Input: part model. Units: mm. Frame: model coordinates. Coordinates: 2 decimals unless noted, no trailing zeros. Order: outer loops, then holes, each group sorted by start corner. A loop starts at its lowest first (then second) coordinate and runs counter-clockwise, first axis right, second up.
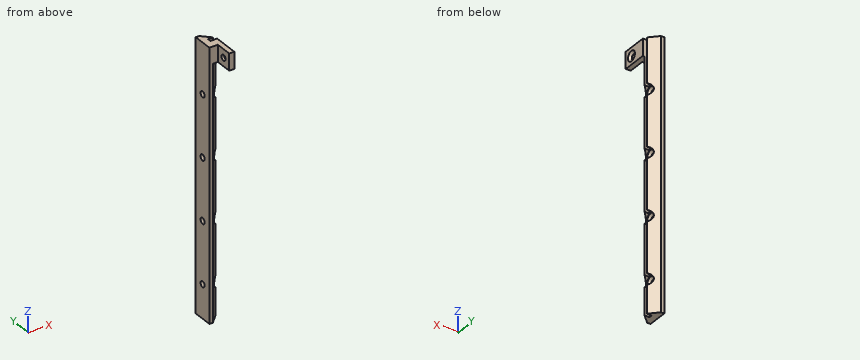
from build123d import *

# Parameters (mm, degrees)
BOSS_EXTRUDE1_DEPTH                            = 75
SKETCH5_R                                      = 1.75
CUT_EXTRUDE1_DEPTH                             = 2
CSK_FOR_0_FLAT_HEAD_MACHINE_SCREW2_D           = 1.778
CSK_FOR_0_FLAT_HEAD_MACHINE_SCREW2_DEPTH       = 3.302
CSK_FOR_0_FLAT_HEAD_MACHINE_SCREW2_CSINK_D     = 3.0226
CSK_FOR_0_FLAT_HEAD_MACHINE_SCREW2_CSINK_ANGLE = 82
CSK_FOR_0_FLAT_HEAD_MACHINE_SCREW2_TIP         = 0.53416509
CHAMFER1_SIZE                                  = 3
SKETCH6_W                                      = 1.5
SKETCH6_H                                      = 5
BOSS_EXTRUDE2_DEPTH                            = 5
CSK_FOR_0_FLAT_HEAD_MACHINE_SCREW1_D           = 1.778
CSK_FOR_0_FLAT_HEAD_MACHINE_SCREW1_DEPTH       = 3.302
CSK_FOR_0_FLAT_HEAD_MACHINE_SCREW1_CSINK_D     = 3.0226
CSK_FOR_0_FLAT_HEAD_MACHINE_SCREW1_CSINK_ANGLE = 82
CSK_FOR_0_FLAT_HEAD_MACHINE_SCREW1_TIP         = 0.53416509


with BuildPart() as part:
    # Sketch1 → Boss-Extrude1 (new body)
    with BuildSketch(Plane.XY):
        Polygon((-2, -3), (2, -3), (2, -0.5), (0, -0.5), (0, 0.5), (2, 0.5), (2, 3), (-2, 3), align=None)
    extrude(amount=BOSS_EXTRUDE1_DEPTH)

    # Sketch5 → Cut-Extrude1 (cut)
    with BuildSketch(Plane(origin=(2, 0, 0), x_dir=(0, 0, -1), z_dir=(1, 0, 0))):
        with Locations((-65, 0)):
            Circle(SKETCH5_R)
        with Locations((-46.66667, 0)):
            Circle(SKETCH5_R)
        with Locations((-28.33334, 0)):
            Circle(SKETCH5_R)
        with Locations((-10.00001, 0)):
            Circle(SKETCH5_R)
    extrude(amount=-CUT_EXTRUDE1_DEPTH, mode=Mode.SUBTRACT)

    # CSK for #0 Flat Head Machine Screw2
    with Locations(Plane(origin=(0, 0, 0), x_dir=(0, 0, -1), z_dir=(1, 0, 0))):
        with Locations((-65, 0), (-10.00001, 0), (-46.66667, 0), (-28.33334, 0)):
            CounterSinkHole(CSK_FOR_0_FLAT_HEAD_MACHINE_SCREW2_D / 2, CSK_FOR_0_FLAT_HEAD_MACHINE_SCREW2_CSINK_D / 2, depth=CSK_FOR_0_FLAT_HEAD_MACHINE_SCREW2_DEPTH, counter_sink_angle=CSK_FOR_0_FLAT_HEAD_MACHINE_SCREW2_CSINK_ANGLE)
            with Locations((0, 0, -(CSK_FOR_0_FLAT_HEAD_MACHINE_SCREW2_DEPTH + CSK_FOR_0_FLAT_HEAD_MACHINE_SCREW2_TIP / 2))):  # 118° drill point
                Cone(0, CSK_FOR_0_FLAT_HEAD_MACHINE_SCREW2_D / 2, CSK_FOR_0_FLAT_HEAD_MACHINE_SCREW2_TIP, mode=Mode.SUBTRACT)

    # Chamfer1
    # the kernel refuses this chamfer: 3 mm, written as the material it takes off along each edge
    with BuildSketch(Plane(origin=(2, -3, -7.715048964), x_dir=(-0.9996219169112968, -0.027495876610586348, 0), z_dir=(0, 0, 1))) as chamfer1_piece_1:
        Polygon((CHAMFER1_SIZE * 0.999621916911, -CHAMFER1_SIZE * 0.0274958766106), (-CHAMFER1_SIZE * 0.0274958766106, -CHAMFER1_SIZE * 0.999621916911), (0, 0), align=None)
    extrude(amount=90.430097928, mode=Mode.SUBTRACT)
    with BuildSketch(Plane(origin=(2, 3, -7.715048964), x_dir=(-0.9996219169112968, 0.027495876610586348, 0), z_dir=(0, 0, 1))) as chamfer1_piece_2:
        Polygon((CHAMFER1_SIZE * 0.999621916911, CHAMFER1_SIZE * 0.0274958766106), (-CHAMFER1_SIZE * 0.0274958766106, CHAMFER1_SIZE * 0.999621916911), (0, 0), align=None)
    extrude(amount=90.430097928, mode=Mode.SUBTRACT)

    # Sketch6 → Boss-Extrude2 (add)
    with BuildSketch(Plane.XY.offset(75)):
        Polygon((-2, 3), (-2, -3), (-1, -3), (1.5, -0.5), (0, -0.5), (0, 0.5), (1.5, 0.5), (-1, 3), align=None)
        Polygon((1.5, -0.5), (-1, -3), (0.5, -3), (2, -3), (2, -0.5), align=None)
        with Locations((1.25, -5.5)):
            Rectangle(SKETCH6_W, SKETCH6_H)
    extrude(amount=BOSS_EXTRUDE2_DEPTH)

    # CSK for #0 Flat Head Machine Screw1
    with Locations(Plane(origin=(2, 0, 0), x_dir=(0, 0, -1), z_dir=(1, 0, 0))):
        with Locations((-77.5, -5.5)):
            CounterSinkHole(CSK_FOR_0_FLAT_HEAD_MACHINE_SCREW1_D / 2, CSK_FOR_0_FLAT_HEAD_MACHINE_SCREW1_CSINK_D / 2, depth=CSK_FOR_0_FLAT_HEAD_MACHINE_SCREW1_DEPTH, counter_sink_angle=CSK_FOR_0_FLAT_HEAD_MACHINE_SCREW1_CSINK_ANGLE)
            with Locations((0, 0, -(CSK_FOR_0_FLAT_HEAD_MACHINE_SCREW1_DEPTH + CSK_FOR_0_FLAT_HEAD_MACHINE_SCREW1_TIP / 2))):  # 118° drill point
                Cone(0, CSK_FOR_0_FLAT_HEAD_MACHINE_SCREW1_D / 2, CSK_FOR_0_FLAT_HEAD_MACHINE_SCREW1_TIP, mode=Mode.SUBTRACT)


solid = part.part
Item 1: Cut plane C-C on z = 36. Return loops of the section in (x, y).
Response values:
outline: (-2, -3) - (-1, -3) - (1.5, -0.5) - (0, -0.5) - (0, 0.5) - (1.5, 0.5) - (-1, 3) - (-2, 3) - close
Item 2: Cut plane B-B on z = 77.5. Return loops of the section in (x, y).
Response values:
outline: (-2, -3) - (0.5, -3) - (0.5, -4.61) - (1.28, -4.61) - (2, -3.99) - (2, -0.5) - (0, -0.5) - (0, 0.5) - (1.5, 0.5) - (-1, 3) - (-2, 3) - close; (0.5, -8) - (2, -8) - (2, -7.01) - (1.28, -6.39) - (0.5, -6.39) - close
Item 3: Pin query (flat end, axial travel): pin 1 Ø1.6 at (x, z) = (1, 72.5) entering from +Y; pin 2 Ø0.8 at (x, z) = (1, 36.5) entering from +Y; pin 3 Ø0.5 at (x, z) = (1, 16.5) entering from -Y; pin 4 Ø1.6 at (y, z) = (0, 28.33) entering from +X. Return the tip coordinate at first contact, or that it passes through.
Response values:
pin 1: stops at y = 1.8
pin 2: stops at y = 1.4
pin 3: stops at y = -1.25
pin 4: passes through
Item 4: Cut plane D-D on z = 65. Return loops of the section in (x, y), then the cut area to 3 significant figures.
Response values:
outline: (-2, -3) - (-1, -3) - (0.25, -1.75) - (0, -1.75) - (0, -1.51) - (-0.72, -0.89) - (-2, -0.89) - close; (-2, 0.89) - (-0.72, 0.89) - (0, 1.51) - (0, 1.75) - (0.25, 1.75) - (-1, 3) - (-2, 3) - close
area: 7.06 mm2
Item 5: Ray query, probe 1 along Z at (x, y) = (-1.2, 0); probe 2 along Y at (x, z) = (-1.1, 65); probe 3 along Y at (x, z) = (0.85, 77.5). Return the intervals inside material, ascending.
Response values:
probe 1: z = 0 to 9.11, 10.89 to 27.44, 29.22 to 45.78, 47.56 to 64.11, 65.89 to 80
probe 2: y = -3 to -0.89, 0.89 to 3
probe 3: y = -8 to -6.39, -4.61 to -0.5, 0.5 to 1.15
Item 6: Cut plane A-A on y = -5.5. Return loops of the section in (x, z).
Response values:
outline: (0.5, 75) - (2, 75) - (2, 75.99) - (1.28, 76.61) - (0.5, 76.61) - close; (0.5, 78.39) - (1.28, 78.39) - (2, 79.01) - (2, 80) - (0.5, 80) - close
